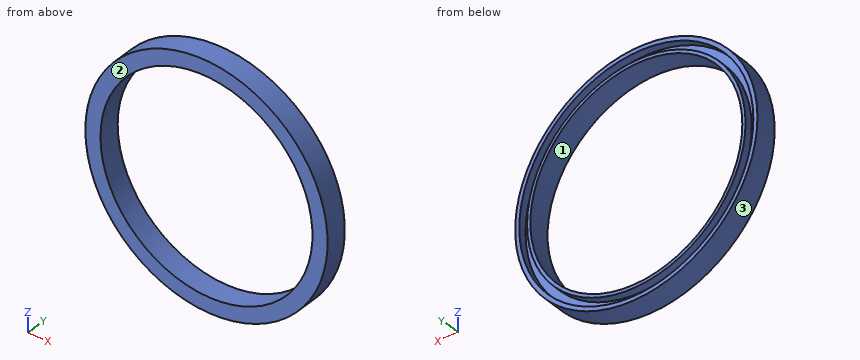
Autodesk Inventor part; units mm, degrees
ref_plane "Work Plane1" through (0, 4.1, 0) normal (0, -1, 0) x (1, 0, 0)
ref_plane "YZ Plane" through (0, 0, 0) normal (1, 0, 0) x (0, 1, 0)
ref_plane "XZ Plane" through (0, 0, 0) normal (0, 1, 0) x (-1, 0, 0)
sketch "Sketch1" plane through (0, 0, 0) normal (0, 1, 0) x (-1, 0, 0)
  circle A0 centre (0, 0) radius 28
  circle A1 centre (0, 0) radius 24.5
  dimension "d0" = 56
  dimension "d5" = 49
extrude "Extrusion2" add sketch "Sketch1" along normal blind 5
sketch "Sketch3" plane through (0, 5, 0) normal (0, 1, 0) x (1, 0, 0)
  circle A0 centre (0, 0) radius 25.25
  circle A1 centre (0, 0) radius 27.05
  dimension "d8" = 50.5
  dimension "d9" = 54.1
extrude "Extrusion3" cut sketch "Sketch3" against normal blind 1.8
ref_plane "Work Plane1" through (0, 4.1, 0) normal (0, -1, 0) x (1, 0, 0)
properties part number "Smaller Cap"
CAD build for the part. Positions are in the model's coordinates, mm. Face numbers are marked on the shaded views. Round coordinates to 2 decimals unless told otherwise and drop trailing zeros. Order: outer loops, then holes, each group sorted by start corner. A loop starts at its lowest first (then second) coordinate and runs counter-clockwise, first axis right, second up. Notation, with made-up numbers: (88, -22.75) - (128, -22.75) arc R12 ccw to (128, -15.75) - close; hole circle Ø9 at (-32, 86). An arc over 180 degrees is marked (long way). Answer in a Markdown table with one row per item. Add a question column.
(1) Drop a flat-ended pin along its axis: pin 1 Ø2 at (x, y) = (4.5, 4) entering from +Z. Give the stop position or say it passes through.
(2) Band-saw the part on A-A on x = 0. List the corners of the cut face in (y, z).
(3) Band-saw the part on D-D on y = 0.8. List the corners of the cut face in (x, z).
(4) Probe L1, parallel to X at y = 4.5, z = 0.5; L2, parallel to Z at x = 0, y = 4.55; L3, parallel to Z at x = 0, y = 3. List the from-to ranges inside material, lowest first. Write a range as [from, to].
(5) Band-saw the part on C-C on y = 4.3. List the corners of the cut face in (x, z).
(6) Band-saw the part on B-B on z = 0. List the corners of the cut face in (x, y), and give its area (3 significant figures).
(7) Mould opens along X. For the marked faces 1, 2 and 3 say: +X half, -X half, draft (parallel to the pull), parting line (faces both ways), or undercut.
Data:
| question | item | result |
|---|---|---|
| 1 | pin 1 | stops at z = 27.78 |
| 2 | outline | (0, -28) - (5, -28) - (5, -27.05) - (3.2, -27.05) - (3.2, -25.25) - (5, -25.25) - (5, -24.5) - (0, -24.5) - close; (0, 24.5) - (5, 24.5) - (5, 25.25) - (3.2, 25.25) - (3.2, 27.05) - (5, 27.05) - (5, 28) - (0, 28) - close |
| 3 | outline | circle Ø56 at (0, 0); hole circle Ø49 at (0, 0) |
| 4 | L1 | x = [-28, -27.05], [-25.25, -24.49], [24.49, 25.25], [27.05, 28] |
| 4 | L2 | z = [-28, -27.05], [-25.25, -24.5], [24.5, 25.25], [27.05, 28] |
| 4 | L3 | z = [-28, -24.5], [24.5, 28] |
| 5 | outline | circle Ø56 at (0, 0); circle Ø50.5 at (0, 0); hole circle Ø54.1 at (0, 0); hole circle Ø49 at (0, 0) |
| 6 | outline | (-28, 0) - (-24.5, 0) - (-24.5, 5) - (-25.25, 5) - (-25.25, 3.2) - (-27.05, 3.2) - (-27.05, 5) - (-28, 5) - close; (24.5, 0) - (28, 0) - (28, 5) - (27.05, 5) - (27.05, 3.2) - (25.25, 3.2) - (25.25, 5) - (24.5, 5) - close |
| 6 | area | 28.5 mm^2 |
| 7 | face 1 | undercut |
| 7 | face 2 | draft |
| 7 | face 3 | parting line |
